Source: three-view drawing plus pictorial views. Frame: mm from the lowest corner of the part. A direction names the side the tool comes from. Give positions to 0.01 mm unless a question says otherwise; leave off trailing zeros. Loops run counter-clockwise (first coordinate to the right, second up) from the corner with the lowest first, then second, coordinate; pieces in that order, holes last. Notation, with made-up numbers: (10.25, -3) - (24.25, -3) arc R25 cw to (24.25, 16) - close; hole circle Ø7 at (67, 53). An arc over 180 degrees is marked (long way). Answer as a JSON object with one key per item and string values.
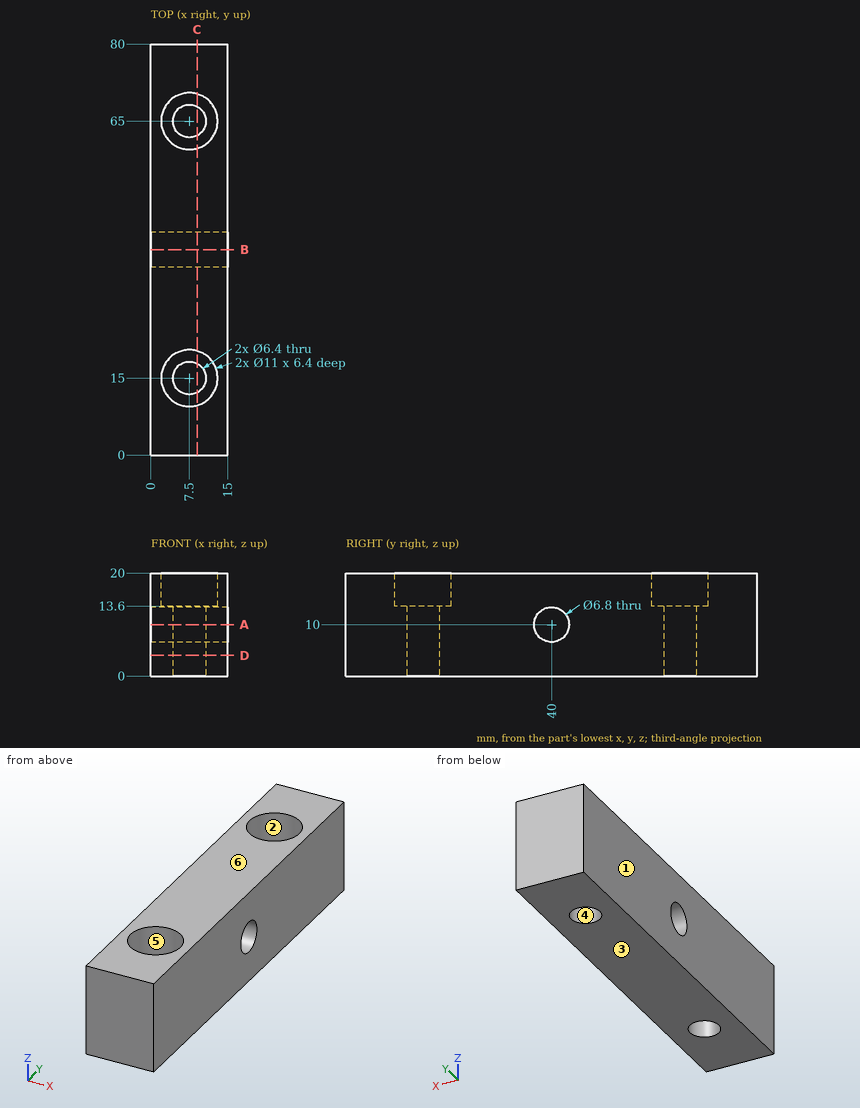
Item 1: Access query for the marked faces 5 and 6. Directions: +Z, -Z, +X, -X, +Y, -Y. A direction counts if a zero-diameter tool reaches every point of the face in a straight line with its end or side. Return the directions, or none.
Geometry check:
{"face 5": "+Z", "face 6": "+Z, +X, -X, +Y, -Y"}
Item 2: Cut plane B-B (y = 40). Return loops of the section in (x, z), then the cut area to 3 significant figures.
Geometry check:
{"outline": "(0, 0) - (15, 0) - (15, 6.6) - (0, 6.6) - close; (0, 13.4) - (15, 13.4) - (15, 20) - (0, 20) - close", "area": "198 mm2"}
Item 3: Material intervals for line 1 (Y direction, x = 7.75, z = 9.75); line 2 (Y direction, x = 7.5, z = 18.5); line 3 (Y direction, x = 7.75, z = 12.25), sorted ascending. Write a range as [from, to].
Geometry check:
{"line 1": "y = [0, 11.81], [18.19, 36.61], [43.39, 61.81], [68.19, 80]", "line 2": "y = [0, 9.5], [20.5, 59.5], [70.5, 80]", "line 3": "y = [0, 11.81], [18.19, 37.45], [42.55, 61.81], [68.19, 80]"}
Item 4: Cut plane A-A (z = 10). Return loops of the section in (x, y).
Geometry check:
{"outline": "(0, 0) - (15, 0) - (15, 36.6) - (0, 36.6) - close; (0, 43.4) - (15, 43.4) - (15, 80) - (0, 80) - close; hole circle Ø6.4 at (7.5, 15); hole circle Ø6.4 at (7.5, 65)"}
Item 5: Cut plane D-D (z = 4). Return loops of the section in (x, y), then the cut area to 3 significant figures.
Geometry check:
{"outline": "(0, 0) - (15, 0) - (15, 80) - (0, 80) - close; hole circle Ø6.4 at (7.5, 15); hole circle Ø6.4 at (7.5, 65)", "area": "1,140 mm2"}
Item 6: Mould query, pull axis X, two halves, no side actions, for the marked faces 1, 2, 3 and 4. Classes: released by +X, released by -X, zero draft, split by the parting line, or undercut.
Geometry check:
{"face 1": "released by -X", "face 2": "undercut", "face 3": "zero draft", "face 4": "undercut"}
Item 7: Cut plane C-C (x = 9). Return loops of the section in (y, z).
Geometry check:
{"outline": "(0, 0) - (12.17, 0) - (12.17, 13.6) - (9.71, 13.6) - (9.71, 20) - (0, 20) - close; (17.83, 0) - (62.17, 0) - (62.17, 13.6) - (59.71, 13.6) - (59.71, 20) - (20.29, 20) - (20.29, 13.6) - (17.83, 13.6) - close; (67.83, 0) - (80, 0) - (80, 20) - (70.29, 20) - (70.29, 13.6) - (67.83, 13.6) - close; hole circle Ø6.8 at (40, 10)"}
